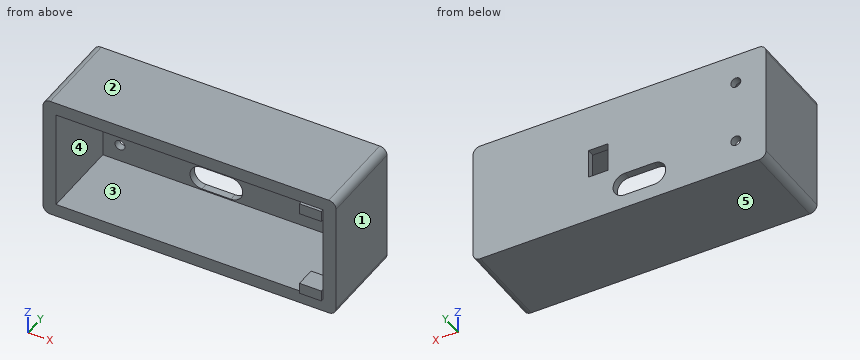
```python
from build123d import *

# Parameters (mm, degrees)
BOSS_EXTRUDE1_DEPTH = 28.2829
BOSS_EXTRUDE2_DEPTH = 2.54
CUT_EXTRUDE1_REACH  = 125.911
SKETCH3_R           = 1.75
SKETCH4_W           = 7.62
SKETCH4_H           = 6.985
BOSS_EXTRUDE3_DEPTH = 3.81
CUT_EXTRUDE2_REACH  = 126.168
SKETCH6_W           = 6.858000092
SKETCH6_H           = 10.16
CUT_EXTRUDE3_REACH  = 126.168


with BuildPart() as part:
    # Sketch1 → Boss-Extrude1 (new body)
    with BuildSketch(Plane(origin=(0, 35.474386892, 0), x_dir=(1, 0, 0), z_dir=(0, 1, 0))):
        with BuildLine():
            Line((-17.013975249, -86.850733206), (80.290024751, -86.850733206))
            ThreePointArc((80.290024751, -86.850733206), (82.086075975, -86.10678443), (82.830024751, -84.310733206))
            Line((82.830024751, -84.310733206), (82.830024751, -46.210733206))
            ThreePointArc((82.830024751, -46.210733206), (82.086075975, -44.414681982), (80.290024751, -43.670733206))
            Line((80.290024751, -43.670733206), (-17.013975249, -43.670733206))
            ThreePointArc((-17.013975249, -43.670733206), (-18.810026474, -44.414681982), (-19.553975249, -46.210733206))
            Line((-19.553975249, -46.210733206), (-19.553975249, -84.310733206))
            ThreePointArc((-19.553975249, -84.310733206), (-18.810026474, -86.10678443), (-17.013975249, -86.850733206))
        make_face()
        Polygon((78.258024751, -82.405733206), (78.258024751, -48.115733206), (-6.791975249, -48.115733206), (-11.171975249, -48.115733206), (-14.981975249, -48.115733206), (-14.981975249, -51.115733206), (-14.981975249, -54.115733206), (-14.981975249, -76.405733206), (-14.981975249, -79.405733206), (-14.981975249, -82.405733206), (-11.171975249, -82.405733206), (-6.791975249, -82.405733206), align=None, mode=Mode.SUBTRACT)
    extrude(amount=BOSS_EXTRUDE1_DEPTH)

    # Sketch2 → Boss-Extrude2 (add)
    with BuildSketch(Plane(origin=(0, 63.757286892, 0), x_dir=(1, 0, 0), z_dir=(0, 1, 0))):
        with BuildLine():
            Line((-17.013975249, -86.850733206), (80.290024751, -86.850733206))
            ThreePointArc((80.290024751, -86.850733206), (82.086075975, -86.10678443), (82.830024751, -84.310733206))
            Line((82.830024751, -84.310733206), (82.830024751, -46.210733206))
            ThreePointArc((82.830024751, -46.210733206), (82.086075975, -44.414681982), (80.290024751, -43.670733206))
            Line((80.290024751, -43.670733206), (-17.013975249, -43.670733206))
            ThreePointArc((-17.013975249, -43.670733206), (-18.810026474, -44.414681982), (-19.553975249, -46.210733206))
            Line((-19.553975249, -46.210733206), (-19.553975249, -84.310733206))
            ThreePointArc((-19.553975249, -84.310733206), (-18.810026474, -86.10678443), (-17.013975249, -86.850733206))
        make_face()
    extrude(amount=BOSS_EXTRUDE2_DEPTH)

    # Sketch3 → Cut-Extrude1 (cut, up to next)
    with BuildSketch(Plane(origin=(0, 66.297286892, 0), x_dir=(1, 0, 0), z_dir=(0, 1, 0)), mode=Mode.PRIVATE) as cut_extrude1_sk1:
        with Locations(Location((-8.981975249, -54.115733206, 0), (0, 0, 270))):
            Circle(SKETCH3_R)
    cut_extrude1_tool1 = extrude(cut_extrude1_sk1.sketch, amount=-CUT_EXTRUDE1_REACH, mode=Mode.PRIVATE) & part.part
    # Sketch3 → Cut-Extrude1 (cut, up to next)
    with BuildSketch(Plane(origin=(0, 66.297286892, 0), x_dir=(1, 0, 0), z_dir=(0, 1, 0)), mode=Mode.PRIVATE) as cut_extrude1_sk2:
        with Locations(Location((-8.981975249, -76.405733206, 0), (0, 0, 270))):
            Circle(SKETCH3_R)
    cut_extrude1_tool2 = extrude(cut_extrude1_sk2.sketch, amount=-CUT_EXTRUDE1_REACH, mode=Mode.PRIVATE) & part.part
    add(cut_extrude1_tool1.solids().sort_by_distance((-8.981975, 66.297287, 54.115733))[0], mode=Mode.SUBTRACT)
    add(cut_extrude1_tool2.solids().sort_by_distance((-8.981975, 66.297287, 76.405733))[0], mode=Mode.SUBTRACT)

    # Sketch4 → Boss-Extrude3 (add)
    with BuildSketch(Plane.XY.offset(48.115733206)):
        with Locations((74.448024751, 37.950886892)):
            Rectangle(SKETCH4_W, SKETCH4_H)
    boss_extrude3 = extrude(amount=BOSS_EXTRUDE3_DEPTH)

    # Mirror1: Boss-Extrude3 across plane
    add(boss_extrude3.mirror(Plane.XY.offset(65.260733206)))

    # Sketch6 → Cut-Extrude2 (cut, up to next)
    with BuildSketch(Plane(origin=(0, 66.297286892, 0), x_dir=(1, 0, 0), z_dir=(0, 1, 0)), mode=Mode.PRIVATE) as cut_extrude2_sk1:
        with Locations((39.039024705, -65.260733206)):
            Rectangle(SKETCH6_W, SKETCH6_H)
    cut_extrude2_tool1 = extrude(cut_extrude2_sk1.sketch, amount=-CUT_EXTRUDE2_REACH, mode=Mode.PRIVATE) & part.part
    add(cut_extrude2_tool1.solids().sort_by_distance((39.039025, 66.297287, 65.260733))[0], mode=Mode.SUBTRACT)

    # Sketch7 → Cut-Extrude3 (cut, up to next)
    with BuildSketch(Plane(origin=(0, 66.297286892, 0), x_dir=(1, 0, 0), z_dir=(0, 1, 0)), mode=Mode.PRIVATE) as cut_extrude3_sk1:
        with BuildLine():
            Line((29.768024751, -56.751733206), (19.608024751, -56.751733206))
            ThreePointArc((19.608024751, -56.751733206), (15.480524751, -52.624233206), (19.608024751, -48.496733206))
            Line((19.608024751, -48.496733206), (29.768024751, -48.496733206))
            ThreePointArc((29.768024751, -48.496733206), (33.895524751, -52.624233206), (29.768024751, -56.751733206))
        make_face()
    cut_extrude3_tool1 = extrude(cut_extrude3_sk1.sketch, amount=-CUT_EXTRUDE3_REACH, mode=Mode.PRIVATE) & part.part
    add(cut_extrude3_tool1.solids().sort_by_distance((24.688025, 66.297287, 52.624233))[0], mode=Mode.SUBTRACT)


solid = part.part
```
Here's how the part is built. I have some questions about the finished solid (model axes, mm). Face numbers are marked on the shaded views. A direction names the side the tool comes from. Coordinates: 2 decimals unless noted, no trailing zeros. Order: outer loops, then holes, each group sorted by start corner. A loop starts at its lowest first (then second) coordinate and runs counter-clockwise, first axis right, second up. Notation, with made-up numbers: M 82,-21 L 138,-21 A19 ccw 138,14 Z; hole C -36.75,56 d8. An arc over 180 degrees is marked long. Answer as a JSON object with one key per item and string values. Group by question number.
(1) Suppose I cut it at C-C, the plane y = 37. Please give me the cut outline in (x, z), then the cut area to 3 significant figures.
(2) If we mould it in two halves opening along Z, with no side actions, what happens to the marked faces 1, 2 and 3? For each: released by +Z, released by -Z, zero draft, split by the parting line, or undercut.
(3) Suppose I cut it at A-A, the plane z = 62. Please give me the cut outline in (x, y), then the cut area to 3 significant figures.
(4) Suppose I cut it at B-B, the plane x = 40.5. Please give me the cut outline in (y, z), then the cut area to 3 significant figures.
(5) For pin 1 (5.5 mm diameter, centred on x = -8.98, z = 54.12, fed in from -Y), with a flat end and sliding along its axis, tell me the tip position at first contact or that it passes through.
(6) I need wall thicknesses on probe 1 along Z at (x, y) = (48, 56.5); probe 2 along X at (y, z) = (48, 64); probe 3 along X at (y, z) = (64.5, 54). Which ranges of each line are inside material? Lowest first, please.
(7) Suppose I cut it at D-D, the plane x = 5.5. Please give me the cut outline in (y, z), then the cut area to 3 significant figures.
(8) Which directions (+Z, -Z, +X, -X, +Y, -Y) give clear straight access to the entire face, cutting with the end or side of a thin tool? Please do the marked faces 4 and 5.
Values found:
{
 "1": {"outline": "M -19.55,46.21 A2.54 ccw -17.01,43.67 L 80.29,43.67 A2.54 ccw 82.83,46.21 L 82.83,84.31 A2.54 ccw 80.29,86.85 L -17.01,86.85 A2.54 ccw -19.55,84.31 Z; hole M -14.98,48.12 L 70.64,48.12 L 70.64,51.93 L 78.26,51.93 L 78.26,78.6 L 70.64,78.6 L 70.64,82.41 L -14.98,82.41 Z", "area": "1,280 mm^2"},
 "2": {"face 1": "zero draft", "face 2": "released by +Z", "face 3": "undercut"},
 "3": {"outline": "M -19.55,35.47 L -14.98,35.47 L -14.98,63.76 L 35.61,63.76 L 35.61,66.3 L -19.55,66.3 Z; M 42.47,63.76 L 78.26,63.76 L 78.26,35.47 L 82.83,35.47 L 82.83,66.3 L 42.47,66.3 Z", "area": "501 mm^2"},
 "4": {"outline": "M 35.47,43.67 L 66.3,43.67 L 66.3,60.18 L 63.76,60.18 L 63.76,48.12 L 35.47,48.12 Z; M 35.47,82.41 L 63.76,82.41 L 63.76,70.34 L 66.3,70.34 L 66.3,86.85 L 35.47,86.85 Z", "area": "335 mm^2"},
 "5": {"pin 1": "stops at y = 63.76"},
 "6": {"probe 1": "z = 43.67 to 48.12, 82.41 to 86.85", "probe 2": "x = -19.55 to -14.98, 78.26 to 82.83", "probe 3": "x = -19.55 to -10.73, -7.24 to 15.72, 33.66 to 82.83"},
 "7": {"outline": "M 35.47,43.67 L 66.3,43.67 L 66.3,86.85 L 35.47,86.85 L 35.47,82.41 L 63.76,82.41 L 63.76,48.12 L 35.47,48.12 Z", "area": "361 mm^2"},
 "8": {"face 4": "-Y", "face 5": "-Z, +X, -X, +Y, -Y"}
}
